Autodesk Inventor part; units mm, degrees
ref_plane "YZ Plane" through (0, 0, 0) normal (1, 0, 0) x (0, 1, 0)
ref_plane "XZ Plane" through (0, 0, 0) normal (0, 1, 0) x (-1, 0, 0)
ref_plane "XY Plane" through (0, 0, 0) normal (0, 0, 1) x (1, 0, 0)
sketch "草图1" plane through (0, 0, 0) normal (0, 0, 1) x (1, 0, 0)
  line L0 (0, 0) -> (300, 0)
  line L1 (300, 0) -> (300, 500)
  line L2 (300, 500) -> (0, 500)
  line L3 (0, 500) -> (0, 0)
  line L4 (150, 500) -> (150, 0)
  circle A0 centre (62.5, 200) radius 20
  circle A1 centre (237.5, 200) radius 20
  dimension "d0" = 300
  dimension "d1" = 500
  dimension "d2" = 40
  dimension "d3" = 200
  dimension "d4" = 175
extrude "拉伸1" add sketch "草图1" along normal blind 20
sketch "草图2" plane through (0, 0, 20) normal (0, 0, 1) x (1, 0, 0)
  line L0 (300, 500) -> (0, 500) construction
  line L1 (0, 500) -> (0, 0) construction
  line L2 (0, 0) -> (300, 0) construction
  line L3 (300, 0) -> (300, 500) construction
  circle A0 centre (62.5, 200) radius 20 construction
  circle A1 centre (237.5, 200) radius 20 construction
  line L4 (300, 500) -> (0, 500)
  line L5 (0, 500) -> (400, 500)
  line L6 (400, 500) -> (400, 300)
  line L7 (400, 300) -> (0, 300)
  line L8 (0, 300) -> (0, 500)
  dimension "d7" = 400
  dimension "d8" = 200
extrude "拉伸2" add sketch "草图2" along normal blind 195
sketch "草图3" plane through (0, 500, 0) normal (0, 1, 0) x (1, 0, 0)
  line L0 (237.5, 53) -> (237.5, -318)
  line L1 (300, 0) -> (0, 0) construction
  line L2 (0, 0) -> (0, -215) construction
  line L3 (400, -215) -> (0, -215) construction
  line L4 (400, -20) -> (400, -215) construction
  line L5 (400, -20) -> (300, -20) construction
  line L6 (300, 0) -> (300, -20) construction
  line L7 (0, -215) -> (400, -215)
  circle A0 centre (237.5, -215) radius 60
  dimension "d11" = 120
extrude "拉伸3" cut sketch "草图3" against normal through all
sketch "草图4" plane through (0, 500, 0) normal (0, 1, 0) x (1, 0, 0)
  line L0 (62.5, 43) -> (62.5, -258)
  arc A0 (297.5, -215) -> (177.5, -215) centre (237.5, -215) ccw construction
  line L1 (0, -215) -> (177.5, -215) construction
  line L2 (0, -20) -> (0, -215) construction
  line L3 (300, -20) -> (0, -20) construction
  line L4 (300, -20) -> (400, -20) construction
  line L5 (400, -20) -> (400, -215) construction
  line L6 (297.5, -215) -> (400, -215) construction
  point P0 (0, 0)
  point P1 (62.5, -80)
  point P2 (62.5, -140)
  dimension "d14" = 60
  dimension "d15" = 60
hole "孔1" at (62.5, 500, 80) at (62.5, 500, 140) direction (0, -1, 0) diameter 25 end through all
sketch "草图5" plane through (0, 0, 0) normal (0, -1, 0) x (1, 0, 0)
  line L0 (0, 0) -> (300, 0) construction
  line L1 (300, 0) -> (300, 20) construction
  line L2 (0, 20) -> (300, 20) construction
  line L3 (0, 0) -> (0, 20) construction
  line L4 (300, 0) -> (0, 0)
  line L5 (150, 0) -> (150, 100)
  line L6 (150, 0) -> (250, 0) construction
  line L7 (300, 20) -> (0, 20) construction
  line L8 (40, 20) -> (60, 20)
  line L9 (60, 20) -> (60, -30)
  line L10 (60, -30) -> (40, -30)
  line L11 (40, -30) -> (40, 20)
  line L12 (260, 20) -> (240, 20)
  line L13 (240, 20) -> (240, -30)
  line L14 (240, -30) -> (260, -30)
  line L15 (260, -30) -> (260, 20)
  dimension "d23" = 100
  dimension "d24" = 90
  dimension "d25" = 300
  dimension "d26" = 20
  dimension "d27" = 50
  dimension "d28" = 180
extrude "拉伸4" add sketch "草图5" against normal blind 10
full round fillet "全圆角1" first side at (60, 3.3333, -20) centre faces at (46.6667, 3.3333, -30) second side at (40, 3.3333, -10)
full round fillet "全圆角2" first side at (260, 3.3333, -20) centre faces at (246.6667, 3.3333, -30) second side at (240, 3.3333, -10)
sketch "草图6" plane through (0, 10, 0) normal (0, 1, 0) x (1, 0, 0)
  arc A0 (260, 20) -> (240, 20) centre (250, 20) ccw
  point P0 (0, 0)
  point P1 (50.1604, 17.9561)
hole "孔2" at (50.1604, 10, -17.9561) at (250, 10, -20) direction (0, -1, 0) diameter 10 end through all
properties part number "主体"
Input: part model. Units: mm. Frame: model coordinates. A direction names the side the tool comes from. Give positions to 0.01 mm unless a question says otherwise; leave off trailing zeros. Order: outer loops, then holes, each group sorted by start corner. A loop starts at its lowest first (then second) coordinate and runs counter-clockwise, first axis right, second up. Notation, with made-up numbers: M -15,10 L 1,10 A5 cw 1,14 Z; hole C 21,46.25 d2. An arc over 180 degrees is marked long. Return JSON: item names as keys, results as strings.
1) Section query D-D on z = 44. Output: boundary loops of the cut face in (x, y), and give its area (3 significant figures).
Taken from the geometry:
{"outline": "M 0,300 L 400,300 L 400,500 L 0,500 Z", "area": "80,000 mm2"}
2) Line query: L1, parallel to Y at x = 62, z = 15; L2, parallel to X at y = 359, z = 140; L3, parallel to Z at x = 250, y = 3.25. Output: solid intervals per line, ascending. Write a range as [from, to].
Taken from the geometry:
{"L1": "y = [0, 180.01], [219.99, 500]", "L2": "x = [0, 50], [75, 400]", "L3": "z = [-30, -25], [-15, 20]"}
3) Contact query for flat-ended pins moving along their axis: pin 1 (11 mm diameter, centred on y = 4, z = -13.5, fed in from -X); pin 2 (6 mm diameter, centred on x = 315.5, z = 84.5, fed in from -Y); pin 3 (9 mm diameter, centred on x = 250, z = -20, fed in from -Y); pin 4 (10 mm diameter, centred on x = 46, z = -9.5, fed in from +Y). Output: stop coordinate, or through.
Taken from the geometry:
{"pin 1": "stops at x = 40", "pin 2": "stops at y = 300", "pin 3": "passes through", "pin 4": "stops at y = 10"}
4) Access query for faces 4 (the face through (148, 152, 20)), 5 (the face through (349, 401, 20)), 6 (the face through (88, 401, 215)), 7 (the face through (50, 10, -11)). Directions: +Z, -Z, +X, -X, +Y, -Y. A direction counts if a zero-diameter tool reaches every point of the face in a straight line with its end or side. Return the directions, or none.
Taken from the geometry:
{"face 4": "+Z, +X, -X, -Y", "face 5": "-Z, +X, +Y, -Y", "face 6": "+Z, +X, -X, +Y, -Y", "face 7": "-Z, +X, -X, +Y"}
5) Section query C-C on x = 116.5. Output: boundary loops of the cut face in (y, z), and give its area (3 significant figures).
Taken from the geometry:
{"outline": "M 0,0 L 500,0 L 500,215 L 300,215 L 300,20 L 0,20 Z", "area": "49,000 mm2"}
6) Section query A-A on y = 200. Output: boundary loops of the cut face in (x, z).
Taken from the geometry:
{"outline": "M 0,0 L 42.5,0 L 42.5,20 L 0,20 Z; M 82.5,0 L 217.5,0 L 217.5,20 L 82.5,20 Z; M 257.5,0 L 300,0 L 300,20 L 257.5,20 Z"}
7) Mould query, pull axis X, two halves, no side actions, for faces 1 (the face through (250, 10, -11)), 2 (the face through (238.819, 401.4, 155.015)), 3 (the face through (0, 358, 106)). Classes: released by +X, released by -X, zero draft, split by the parting line, or undercut.
Taken from the geometry:
{"face 1": "zero draft", "face 2": "undercut", "face 3": "released by -X"}
8) Section query B-B on z = 140. Output: boundary loops of the cut face in (x, y).
Taken from the geometry:
{"outline": "M 0,300 L 50,300 L 50,500 L 0,500 Z; M 75,300 L 400,300 L 400,500 L 75,500 Z"}
